The model under review builds one solid part; all positions refer to its coordinate system, in mm. Face numbers are marked on the shaded views. A direction names the side the tool comes from. Coordinates: 2 decimals unless noted, no trailing zeros. Order: outer loops, then holes, each group sorted by start corner. A loop starts at its lowest first (then second) coordinate and runs counter-clockwise, first axis right, second up. Notation, with made-up numbers: (9, 80.5) -> (27, 80.5) arc R23 cw to (27, 119.5) -> close; hole circle Ø8 at (76.5, 57). An arc over 180 degrees is marked (long way). Use one line per item in the form item = value. Start each with the question number.
(1) Take a section at A-A (z = 24.7). State the section outline as (x, y) points, then the cut area to 3 significant figures.
(2) Wall thickness on line 1 along Z through (x, y) = (36.65, 6.5); line 2 along Z through (x, y) = (43.5, 8.5); line 3 along X through (y, z) = (11.5, 22.5): over which ranges is each line inside the solid? List them lowest first.
(3) Mouldability with a two-part tool opening along Z and no side actions: class the marked faces 3, 4, 5 and 6 as +Z half, -Z half, draft (parallel to the pull), parting line (faces both ways), or undercut.
(4) Take a section at B-B (z = 51.5). State the section outline as (x, y) points, then the cut area to 3 significant figures.
(5) Take a section at C-C (x = 41). State the section outline as (y, z) points.
(6) Take a section at D-D (y = 1.25). State the section outline as (x, z) points.
(7) For the marked faces 1 and 2, list the 3-axis set-ups (+Z, -Z, +X, -X, +Y, -Y) from which the entire face can be reached by the end or side of a thin tool; tool diameter is ignored.
(8) Insertion check: pin 1 Ø1.6 at (y, z) = (6.5, 24.7) entering from -X; pin 2 Ø2.5 at (y, z) = (6.5, 30.3) entering from +X; pin 3 Ø6 at (x, z) = (42, 9) entering from +Y. Each pin has a flat end and moves straight along its axis. Give the tip position at first contact, or say it passes through.
```python
from build123d import *

# Parameters (mm, degrees)
SKETCH1_W           = 70
SKETCH1_H           = 3
BOSS_EXTRUDE1_DEPTH = 55
SKETCH2_W           = 70
SKETCH2_H           = 2.5
BOSS_EXTRUDE2_DEPTH = 22.8
SKETCH5_R           = 3.5
CUT_EXTRUDE1_DEPTH  = 84.8
SKETCH6_W           = 16
SKETCH6_H           = 11.6
SKETCH6_W_2         = 15
BOSS_EXTRUDE7_DEPTH = 22.8
SKETCH7_R           = 1
CUT_EXTRUDE2_DEPTH  = 8
SKETCH8_R           = 1
CUT_EXTRUDE3_DEPTH  = 8
FILLET1_R           = 5
SKETCH9_W           = 14.084433838
SKETCH9_H           = 7
CUT_EXTRUDE4_DEPTH  = 66
SKETCH10_R          = 1.25
BOSS_EXTRUDE8_DEPTH = 55
SKETCH11_W          = 19.22261198
SKETCH11_H          = 30.8
CUT_EXTRUDE5_DEPTH  = 35
SKETCH12_W          = 30.8
SKETCH12_H          = 25.8
SKETCH12_R          = 1
BOSS_EXTRUDE9_DEPTH = 3
CUT_EXTRUDE6_DEPTH  = 96
SKETCH14_W          = 89.735472453
SKETCH14_H          = 73.087764116
CUT_EXTRUDE7_DEPTH  = 96


with BuildPart() as part:
    # Sketch1 → Boss-Extrude1 (new body)
    with BuildSketch(Plane.XY):
        Rectangle(SKETCH1_W, SKETCH1_H)
    extrude(amount=BOSS_EXTRUDE1_DEPTH)

    # Sketch2 → Boss-Extrude2 (add)
    with BuildSketch(Plane(origin=(0, 1.5, 0), x_dir=(1, 0, 0), z_dir=(0, 1, 0))):
        with Locations((0, -1.25)):
            Rectangle(SKETCH2_W, SKETCH2_H)
        with Locations((0, -53.75)):
            Rectangle(SKETCH2_W, SKETCH2_H)
    extrude(amount=BOSS_EXTRUDE2_DEPTH)

    # Sketch5 → Cut-Extrude1 (cut)
    with BuildSketch(Plane.XY.offset(55)):
        with Locations((-24, 11.4)):
            Circle(SKETCH5_R)
    extrude(amount=-CUT_EXTRUDE1_DEPTH, mode=Mode.SUBTRACT)

    # Sketch6 → Boss-Extrude7 (add)
    with BuildSketch(Plane(origin=(0, 24.3, 0), x_dir=(1, 0, 0), z_dir=(0, 1, 0))):
        with Locations((-7, -27.5)):
            Rectangle(SKETCH6_W, SKETCH6_H)
        with Locations((27.5, -27.5)):
            Rectangle(SKETCH6_W_2, SKETCH6_H)
    extrude(amount=-BOSS_EXTRUDE7_DEPTH)

    # Sketch7 → Cut-Extrude2 (cut)
    with BuildSketch(Plane(origin=(0, 24.3, 0), x_dir=(1, 0, 0), z_dir=(0, 1, 0))):
        with Locations((-12, -24.7)):
            Circle(SKETCH7_R)
        with Locations((23, -30.3)):
            Circle(SKETCH7_R)
        with Locations((-2, -24.7)):
            Circle(SKETCH7_R)
        with Locations((-2, -30.3)):
            Circle(SKETCH7_R)
        with Locations((-12, -30.3)):
            Circle(SKETCH7_R)
        with Locations((23, -24.7)):
            Circle(SKETCH7_R)
        with Locations((32, -24.7)):
            Circle(SKETCH7_R)
        with Locations((32, -30.3)):
            Circle(SKETCH7_R)
    extrude(amount=-CUT_EXTRUDE2_DEPTH, mode=Mode.SUBTRACT)

    # Sketch8 → Cut-Extrude3 (cut)
    with BuildSketch(Plane(origin=(35, 0, 0), x_dir=(0, 0, -1), z_dir=(1, 0, 0))):
        with Locations((-24.7, 19.3)):
            Circle(SKETCH8_R)
        with Locations((-30.3, 19.3)):
            Circle(SKETCH8_R)
        with Locations((-24.7, 6.5)):
            Circle(SKETCH8_R)
        with Locations((-30.3, 6.5)):
            Circle(SKETCH8_R)
    extrude(amount=-CUT_EXTRUDE3_DEPTH, mode=Mode.SUBTRACT)

    # Fillet1
    fillet1_edges = [part.edges().sort_by_distance(p)[0] for p in [
        (1, 1.5, 27.5),
        (-15, 1.5, 27.5),
        (20, 1.5, 27.5),
    ]]
    fillet(fillet1_edges, radius=FILLET1_R)

    # Sketch9 → Cut-Extrude4 (cut)
    with BuildSketch(Plane.XY.offset(55)):
        with Locations((-31.042216919, 11.4)):
            Rectangle(SKETCH9_W, SKETCH9_H)
    extrude(amount=-CUT_EXTRUDE4_DEPTH, mode=Mode.SUBTRACT)

    # Sketch10 → Boss-Extrude8 (add)
    with BuildSketch(Plane.XY.offset(55)):
        with BuildLine():
            Line((35, 24.3), (49.731333151, 10.422398492))
            ThreePointArc((49.731333151, 10.422398492), (51.413444846, 2.85486244), (45, -1.5))
            Line((45, -1.5), (35, -1.5))
            Line((35, -1.5), (35, 24.3))
        make_face()
        with Locations((45, 5.4)):
            Circle(SKETCH10_R, mode=Mode.SUBTRACT)
    extrude(amount=-BOSS_EXTRUDE8_DEPTH)

    # Sketch11 → Cut-Extrude5 (cut)
    with BuildSketch(Plane.XZ.offset(1.5)):
        with Locations((44.61130599, 27.5)):
            Rectangle(SKETCH11_W, SKETCH11_H)
    extrude(amount=-CUT_EXTRUDE5_DEPTH, mode=Mode.SUBTRACT)

    # Sketch12 → Boss-Extrude9 (add)
    with BuildSketch(Plane(origin=(35, 0, 0), x_dir=(0, 0, -1), z_dir=(1, 0, 0))):
        with Locations((-27.5, 11.4)):
            Rectangle(SKETCH12_W, SKETCH12_H)
        with Locations((-30.3, 19.3)):
            Circle(SKETCH12_R, mode=Mode.SUBTRACT)
        with Locations((-30.3, 6.5)):
            Circle(SKETCH12_R, mode=Mode.SUBTRACT)
        with Locations((-24.7, 6.5)):
            Circle(SKETCH12_R, mode=Mode.SUBTRACT)
        with Locations((-24.7, 19.3)):
            Circle(SKETCH12_R, mode=Mode.SUBTRACT)
    extrude(amount=BOSS_EXTRUDE9_DEPTH)

    # Sketch13 → Cut-Extrude6 (cut)
    with BuildSketch(Plane(origin=(0, 0, 0), x_dir=(-1, 0, 0), z_dir=(0, 0, -1))):
        Polygon((-35, 24.3), (-38, 21.473860363), (-40.585256697, 23.898774346), (-37.538023225, 25.511318129), align=None)
    extrude(amount=-CUT_EXTRUDE6_DEPTH, mode=Mode.SUBTRACT)

    # Sketch14 → Cut-Extrude7 (cut)
    with BuildSketch(Plane(origin=(0, 24.3, 0), x_dir=(1, 0, 0), z_dir=(0, 1, 0))):
        with Locations((-9.867736226, -18.456117942)):
            Rectangle(SKETCH14_W, SKETCH14_H)
    extrude(amount=-CUT_EXTRUDE7_DEPTH, mode=Mode.SUBTRACT)


solid = part.part
```
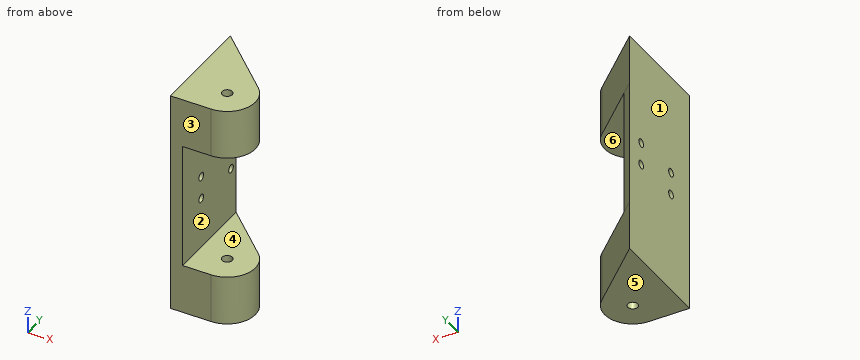
Findings:
q1.outline = (35, -1.5) -> (38, -1.5) -> (38, 5.5) -> (35, 5.5) -> close; (35, 7.5) -> (38, 7.5) -> (38, 18.3) -> (35, 18.3) -> close; (35, 20.3) -> (38, 20.3) -> (38, 21.47) -> (35, 24.3) -> close
q1.area = 61.2 mm²
q2.line_1 = 0 to 23.7, 25.7 to 29.3, 31.3 to 55
q2.line_2 = 0 to 12.1, 42.9 to 55
q2.line_3 = 35 to 38
q3.face_3 = draft
q3.face_4 = undercut
q3.face_5 = -Z half
q3.face_6 = undercut
q4.outline = (35, -1.5) -> (45, -1.5) arc R6.9 ccw to (49.73, 10.42) -> (35, 24.3) -> close; hole circle Ø2.5 at (45, 5.4)
q4.area = 285 mm²
q5.outline = (-1.5, 0) -> (18.65, 0) -> (18.65, 12.1) -> (-1.5, 12.1) -> close; (-1.5, 42.9) -> (18.65, 42.9) -> (18.65, 55) -> (-1.5, 55) -> close
q6.outline = (35, 0) -> (50.51, 0) -> (50.51, 12.1) -> (38, 12.1) -> (38, 42.9) -> (50.51, 42.9) -> (50.51, 55) -> (35, 55) -> close
q7.face_1 = +Z, -Z, -X, +Y, -Y
q7.face_2 = +X, +Y, -Y
q8.pin_1 = through
q8.pin_2 = 38
q8.pin_3 = 20.53
